Autodesk Inventor part; units mm, degrees
ref_plane "YZ Plane" through (0, 0, 0) normal (1, 0, 0) x (0, 1, 0)
ref_plane "XZ Plane" through (0, 0, 0) normal (0, 1, 0) x (-1, 0, 0)
ref_plane "XY Plane" through (0, 0, 0) normal (0, 0, 1) x (1, 0, 0)
ref_plane "Work Plane1" through (0, 0, 0) normal (0, 0, 1) x (1, 0, 0)
sketch "Sketch1" plane through (0, 0, 0) normal (0, 0, 1) x (1, 0, 0)
  arc A0 (5.9062, 3.651) -> (7.7035, 4.7619) centre (6.8048, 4.2064) ccw
  arc A1 (5.9062, 3.651) -> (2.5768, 6.4477) centre (0, 0) ccw
  arc A2 (3.3608, 8.4097) -> (2.5768, 6.4477) centre (2.9688, 7.4287) ccw
  arc A3 (7.7035, 4.7619) -> (3.3608, 8.4097) centre (0, 0) ccw
  arc A4 (2.5768, -6.4477) -> (3.3608, -8.4097) centre (2.9688, -7.4287) ccw
  arc A5 (2.5768, -6.4477) -> (5.9062, -3.651) centre (0, 0) ccw
  arc A6 (7.7035, -4.7619) -> (5.9062, -3.651) centre (6.8048, -4.2064) ccw
  arc A7 (3.3608, -8.4097) -> (7.7035, -4.7619) centre (0, 0) ccw
  arc A8 (-2.5553, 6.4563) -> (-3.3328, 8.4209) centre (-2.9441, 7.4386) ccw
  arc A9 (-2.5553, 6.4563) -> (-5.9062, 3.651) centre (0, 0) ccw
  arc A10 (-7.7035, 4.7619) -> (-5.9062, 3.651) centre (-6.8048, 4.2064) ccw
  arc A11 (-3.3328, 8.4209) -> (-7.7035, 4.7619) centre (0, 0) ccw
  arc A12 (-5.9062, -3.651) -> (-7.7035, -4.7619) centre (-6.8048, -4.2064) ccw
  arc A13 (-5.9062, -3.651) -> (-2.5553, -6.4563) centre (0, 0) ccw
  arc A14 (-3.3328, -8.4209) -> (-2.5553, -6.4563) centre (-2.9441, -7.4386) ccw
  arc A15 (-7.7035, -4.7619) -> (-3.3328, -8.4209) centre (0, 0) ccw
  circle A16 centre (0.0124, -10.65) radius 1.15
  circle A17 centre (8, 0) radius 1.0564
  circle A18 centre (-8, 0) radius 1.0564
  circle A19 centre (0, 0) radius 5
  circle A20 centre (0, 0) radius 13.7
  line L0 (0, 14.375) -> (-17.375, 14.375)
  line L1 (-17.375, 14.375) -> (-17.375, -14.375)
  line L2 (-17.375, -14.375) -> (0, -14.375)
  circle A21 centre (0, 0) radius 5.15
  arc A22 (5.4809, 3.3881) -> (8.1288, 5.0248) centre (6.8048, 4.2064) ccw
  arc A23 (5.4809, 3.3881) -> (2.3912, 5.9835) centre (0, 0) ccw
  arc A24 (3.5464, 8.874) -> (2.3912, 5.9835) centre (2.9688, 7.4287) ccw
  arc A25 (8.1288, 5.0248) -> (3.5464, 8.874) centre (0, 0) ccw
  arc A26 (8.1288, -5.0248) -> (5.4809, -3.3881) centre (6.8048, -4.2064) ccw
  arc A27 (2.3912, -5.9835) -> (5.4809, -3.3881) centre (0, 0) ccw
  arc A28 (2.3912, -5.9835) -> (3.5464, -8.874) centre (2.9688, -7.4287) ccw
  arc A29 (3.5464, -8.874) -> (8.1288, -5.0248) centre (0, 0) ccw
  circle A30 centre (0.0124, -10.65) radius 1.65
  arc A31 (-5.4809, -3.3881) -> (-2.3713, -5.9914) centre (0, 0) ccw
  arc A32 (-5.4809, -3.3881) -> (-8.1288, -5.0248) centre (-6.8048, -4.2064) ccw
  arc A33 (-8.1288, -5.0248) -> (-3.5168, -8.8858) centre (0, 0) ccw
  arc A34 (-3.5168, -8.8858) -> (-2.3713, -5.9914) centre (-2.9441, -7.4386) ccw
  arc A35 (-2.3713, 5.9914) -> (-5.4809, 3.3881) centre (0, 0) ccw
  arc A36 (-2.3713, 5.9914) -> (-3.5168, 8.8858) centre (-2.9441, 7.4386) ccw
  arc A37 (-3.5168, 8.8858) -> (-8.1288, 5.0248) centre (0, 0) ccw
  arc A38 (-8.1288, 5.0248) -> (-5.4809, 3.3881) centre (-6.8048, 4.2064) ccw
  circle A39 centre (-14.375, -11.375) radius 1.75
  circle A40 centre (-14.375, 11.375) radius 1.75
  arc A41 (0, 13.7) -> (0, -13.7) centre (0, 0) ccw
  line L3 (0, -14.375) -> (0, -13.7)
  line L4 (0, 13.7) -> (0, 14.375)
  line L5 (16.125, 8.6145) -> (16.125, -8.7895)
  line L6 (0, -14.375) -> (16.125, -14.375)
  line L7 (16.125, -14.375) -> (16.125, 14.375)
  line L8 (16.125, 14.375) -> (0, 14.375)
  line L9 (0, 14.375) -> (0, -14.375)
  point P0 (0, 0)
  dimension "d0" = 0.15
  dimension "d1" = 0.5
  dimension "d2" = 0.5
  dimension "d3" = 0.5
  dimension "d4" = 0.5
  dimension "d5" = 0.5
extrude "Extrusion1" add sketch "Sketch1" along normal blind 1.5 contours L9 A21 A20 A30 | A30 L9 A20 A21 | L3 L2 L1 L0 L4 A20 | A20 L4 L8 L7 L5 L6 L3 | A39 | A40
sketch "Sketch2" plane through (0, 0, 1.5) normal (0, 0, 1) x (1, 0, 0)
  line L0 (-17.375, 14.375) -> (-17.375, -14.375)
  line L1 (-17.375, -14.375) -> (16.125, -14.375)
  line L2 (16.125, -14.375) -> (16.125, 14.375)
  line L3 (16.125, 14.375) -> (-17.375, 14.375)
  circle A0 centre (8, 0) radius 1.0564
  circle A1 centre (-8, 0) radius 1.0564
  circle A2 centre (0, 0) radius 5.15
  arc A3 (5.4809, 3.3881) -> (2.3912, 5.9835) centre (0, 0) ccw
  arc A4 (3.5464, 8.874) -> (2.3912, 5.9835) centre (2.9688, 7.4287) ccw
  arc A5 (8.1288, 5.0248) -> (3.5464, 8.874) centre (0, 0) ccw
  arc A6 (5.4809, 3.3881) -> (8.1288, 5.0248) centre (6.8048, 4.2064) ccw
  arc A7 (2.3912, -5.9835) -> (5.4809, -3.3881) centre (0, 0) ccw
  arc A8 (8.1288, -5.0248) -> (5.4809, -3.3881) centre (6.8048, -4.2064) ccw
  arc A9 (3.5464, -8.874) -> (8.1288, -5.0248) centre (0, 0) ccw
  arc A10 (2.3912, -5.9835) -> (3.5464, -8.874) centre (2.9688, -7.4287) ccw
  circle A11 centre (0.0124, -10.65) radius 1.65
  arc A12 (-5.4809, -3.3881) -> (-8.1288, -5.0248) centre (-6.8048, -4.2064) ccw
  arc A13 (-5.4809, -3.3881) -> (-2.3713, -5.9914) centre (0, 0) ccw
  arc A14 (-3.5168, -8.8858) -> (-2.3713, -5.9914) centre (-2.9441, -7.4386) ccw
  arc A15 (-8.1288, -5.0248) -> (-3.5168, -8.8858) centre (0, 0) ccw
  arc A16 (-2.3713, 5.9914) -> (-3.5168, 8.8858) centre (-2.9441, 7.4386) ccw
  arc A17 (-2.3713, 5.9914) -> (-5.4809, 3.3881) centre (0, 0) ccw
  arc A18 (-8.1288, 5.0248) -> (-5.4809, 3.3881) centre (-6.8048, 4.2064) ccw
  arc A19 (-3.5168, 8.8858) -> (-8.1288, 5.0248) centre (0, 0) ccw
  arc A20 (8.1288, -5.0248) -> (5.4809, -3.3881) centre (6.8048, -4.2064) ccw
  line L4 (8.3613, -4.2064) -> (8.3613, -14.375)
  line L5 (-17.375, -14.375) -> (16.125, -14.375)
  arc A21 (-5.4809, -3.3881) -> (-8.1288, -5.0248) centre (-6.8048, -4.2064) ccw
  line L6 (-8.3613, -4.2064) -> (-8.3613, -14.375)
  arc A22 (2.3912, -5.9835) -> (3.5464, -8.874) centre (2.9688, -7.4287) ccw
  line L7 (1.6624, -6.5827) -> (-1.6441, -6.5827)
  arc A23 (-3.5168, -8.8858) -> (-2.3713, -5.9914) centre (-2.9441, -7.4386) ccw
  point P0 (0, 0)
extrude "Extrusion2" add sketch "Sketch2" along normal blind 1.5 contours L3 L2 L1 L4 A8 A7 A10 L7 A14 A13 A12 L6 L0
sketch "Sketch3" plane through (0, 0, 3) normal (0, 0, 1) x (1, 0, 0)
  circle A0 centre (0, 0) radius 6.75
  line L0 (-17.375, -14.375) -> (-8.3613, -14.375)
  line L1 (-8.3613, -14.375) -> (-8.3613, -4.2064)
  arc A1 (-5.4809, -3.3881) -> (-8.3613, -4.2064) centre (-6.8048, -4.2064) ccw
  arc A2 (-5.4809, -3.3881) -> (-2.3713, -5.9914) centre (0, 0) ccw
  arc A3 (-1.6441, -6.5827) -> (-2.3713, -5.9914) centre (-2.9441, -7.4386) ccw
  line L2 (-1.6441, -6.5827) -> (1.6624, -6.5827)
  arc A4 (2.3912, -5.9835) -> (1.6624, -6.5827) centre (2.9688, -7.4287) ccw
  arc A5 (2.3912, -5.9835) -> (5.4809, -3.3881) centre (0, 0) ccw
  arc A6 (8.3613, -4.2064) -> (5.4809, -3.3881) centre (6.8048, -4.2064) ccw
  line L3 (8.3613, -4.2064) -> (8.3613, -14.375)
  line L4 (8.3613, -14.375) -> (16.125, -14.375)
  line L5 (16.125, -14.375) -> (16.125, 14.375)
  line L6 (16.125, 14.375) -> (-17.375, 14.375)
  line L7 (-17.375, 14.375) -> (-17.375, -14.375)
  circle A7 centre (8, 0) radius 1.0564
  circle A8 centre (-8, 0) radius 1.0564
  arc A9 (-2.3713, 5.9914) -> (-5.4809, 3.3881) centre (0, 0) ccw
  arc A10 (-8.1288, 5.0248) -> (-5.4809, 3.3881) centre (-6.8048, 4.2064) ccw
  arc A11 (-3.5168, 8.8858) -> (-8.1288, 5.0248) centre (0, 0) ccw
  arc A12 (-2.3713, 5.9914) -> (-3.5168, 8.8858) centre (-2.9441, 7.4386) ccw
  arc A13 (5.4809, 3.3881) -> (8.1288, 5.0248) centre (6.8048, 4.2064) ccw
  arc A14 (5.4809, 3.3881) -> (2.3912, 5.9835) centre (0, 0) ccw
  arc A15 (3.5464, 8.874) -> (2.3912, 5.9835) centre (2.9688, 7.4287) ccw
  arc A16 (8.1288, 5.0248) -> (3.5464, 8.874) centre (0, 0) ccw
  circle A17 centre (0, 0) radius 5.15
  circle A18 centre (8, 0) radius 2.5
  circle A19 centre (-8, 0) radius 2.5
  line L8 (2.9688, 8.9852) -> (-2.9441, 8.9852)
  line L9 (2.9688, 8.9852) -> (8.8817, 8.9852) construction
  arc A20 (-8.1288, 5.0248) -> (-5.4809, 3.3881) centre (-6.8048, 4.2064) ccw
  line L10 (-8.3613, 4.2064) -> (-8.3613, -4.2064)
  arc A21 (-5.4809, -3.3881) -> (-8.1288, -5.0248) centre (-6.8048, -4.2064) ccw
  arc A22 (5.4809, 3.3881) -> (8.1288, 5.0248) centre (6.8048, 4.2064) ccw
  line L11 (8.3613, 4.2064) -> (8.3613, -4.2064)
  point P0 (0, 0)
  point P1 (-8.3613, -2.4738)
  point P2 (-8.3613, 2.4738)
  point P3 (-2.7693, 8.9852)
  point P4 (8.3613, 2.4738)
  point P5 (8.3613, -2.4738)
  dimension "d10" = 5
  dimension "d11" = 5
  dimension "d12" = 180
extrude "Extrusion3" add sketch "Sketch3" along normal blind 1.5 contours L11 A13 A16 A15 L8 A12 A11 A10 L10 A19 L1 L0 L7 L6 L5 L4 L3 A18
sketch "Sketch4" plane through (0, 0, 4.5) normal (0, 0, 1) x (1, 0, 0)
  line L0 (16.125, -14.375) -> (16.125, 14.375)
  line L1 (-17.375, -14.375) -> (16.125, -14.375)
  line L2 (16.125, 14.375) -> (12.625, 14.375)
  line L3 (12.625, -14.375) -> (16.125, -14.375)
  line L4 (16.125, -14.375) -> (16.125, 14.375)
  circle A0 centre (13.125, 11.375) radius 3
  circle A1 centre (13.125, -11.375) radius 3
  circle A2 centre (-14.375, -11.375) radius 3
  circle A3 centre (-14.375, 11.375) radius 3
  line L5 (-8.3613, -14.375) -> (-8.3613, -2.4738)
  arc A4 (-8.3613, 2.4738) -> (-8.3613, -2.4738) centre (-8, 0) ccw
  line L6 (-8.3613, 2.4738) -> (-8.3613, 4.2064)
  arc A5 (-8.1288, 5.0248) -> (-8.3613, 4.2064) centre (-6.8048, 4.2064) ccw
  arc A6 (-3.5168, 8.8858) -> (-8.1288, 5.0248) centre (0, 0) ccw
  arc A7 (-2.7693, 8.9852) -> (-3.5168, 8.8858) centre (-2.9441, 7.4386) ccw
  line L7 (-2.7693, 8.9852) -> (2.9688, 8.9852)
  arc A8 (3.5464, 8.874) -> (2.9688, 8.9852) centre (2.9688, 7.4287) ccw
  arc A9 (8.1288, 5.0248) -> (3.5464, 8.874) centre (0, 0) ccw
  arc A10 (8.3613, 4.2064) -> (8.1288, 5.0248) centre (6.8048, 4.2064) ccw
  line L8 (8.3613, 4.2064) -> (8.3613, 2.4738)
  arc A11 (8.3613, -2.4738) -> (8.3613, 2.4738) centre (8, 0) ccw
  line L9 (8.3613, -2.4738) -> (8.3613, -14.375)
  line L10 (8.3613, -14.375) -> (16.125, -14.375)
  line L11 (16.125, -14.375) -> (16.125, 14.375)
  line L12 (16.125, 14.375) -> (-17.375, 14.375)
  line L13 (-17.375, 14.375) -> (-17.375, -14.375)
  line L14 (-17.375, -14.375) -> (-8.3613, -14.375)
  point P0 (0, 0)
  dimension "d16" = 6
  dimension "d17" = 6
  dimension "d18" = 6
  dimension "d19" = 6
hole "Hole1" at (-14.375, -11.375, 4.5) at (-14.375, 11.375, 4.5) direction (0, 0, -1) diameter 2.9 end through all countersink diameter 5 countersink angle 90
sketch "Sketch6" plane through (16.125, -14.375, 0) normal (1, 0, 0) x (0, 0, -1)
  line L0 (0, 0) -> (0, 28.75)
  line L1 (0, 28.75) -> (-4.5, 28.75)
  line L2 (-4.5, 0) -> (-4.5, 28.75)
  line L3 (0, 0) -> (-4.5, 0)
  line L4 (0, 28.75) -> (-4.5, 28.75)
  line L5 (-4.5, 28.75) -> (-4.5, 24.25)
  line L6 (-4.5, 24.25) -> (0, 24.25)
  line L7 (0, 24.25) -> (0, 28.75)
  line L8 (0, 0) -> (-4.5, 0)
  line L9 (-4.5, 0) -> (-4.5, 4.5)
  line L10 (-4.5, 4.5) -> (0, 4.5)
  line L11 (0, 4.5) -> (0, 0)
  line L12 (-4.5, 24.25) -> (0, 28.75)
  line L13 (-4.5, 28.75) -> (0, 24.25)
  line L14 (0, 0) -> (-4.5, 0)
  line L15 (0, 4.5) -> (-4.5, 0)
  line L16 (0, 0) -> (-4.5, 4.5)
  point P0 (0, 14.375)
  point P1 (-2.25, 26.5)
  point P2 (-2.25, 2.25)
  dimension "d34" = 4.5
  dimension "d35" = 4.5
  dimension "d36" = 4.5
  dimension "d37" = 4.5
hole "Hole3" at (16.125, 12.125, 2.25) at (16.125, -12.125, 2.25) direction (-1, 0, 0) diameter 3 depth 3.5 counterbore diameter 3.5 counterbore depth 1.5
properties part number "right_motor_front_mount" material "Nylon 6/6"
Check sheet for the modelled part. Datum: model origin and axes. Units: mm. A direction names the side the tool comes from. Give positions to 0.01 mm unless a question says otherwise; leave off trailing zeros. Write each loop counter-clockwise with the first axis right and the second up, starting at its lowest first coordinate (ties: lowest second). Pieces come first, ordered by that corner, then holes. Notation, with made-up numbers: M 70.5,24 L 121.5,24 A18 ccw 121.5,41 Z; hole C 22,9.25 d6. An arc over 180 degrees is marked long. Use one line per item in the form item = value.
(1) Section check B-B on x = 0. Record the boundary of the cut face in (y, z) (3 decimals).
Answer block:
outline = M -14.375,0 L -12.3,0 L -12.3,1.5 L -14.375,1.5 Z; M -9,0 L -5.15,0 L -5.15,3 L -6.583,3 L -6.583,1.5 L -9,1.5 Z; M 5.15,0 L 14.375,0 L 14.375,4.5 L 8.985,4.5 L 8.985,3 L 5.15,3 Z
(2) Section check C-C on z = 2.25. State how many separate pieces and enclosed holes the cut face has, plus the area to 3 significant figures.
Answer block:
separate_pieces = 1
enclosed_holes = 7
area = 628 mm2
(3) Draft check along Z on faces 1 (the cylindrical face through (15.36, -13.86, 2.48)), 2 (the flat face through (-2, 5, 3)), 3 (the flat face through (16.125, 0, 2)). Enter one of: pulls with the +Z half, pulls with the -Z half, needs draft (parallel to the pull), parting line crosses it, or undercut.
Answer block:
face_1 = undercut
face_2 = pulls with the +Z half
face_3 = needs draft
(4) Material ranges on line 1 along Y through (x, z) = (-14.5, 1.35) (3 decimals); line 2 along X through (y, z) = (-11.5, 3.2) (3 decimals); line 3 along X through (y, z) = (-7.75, 2.95) (3 decimals), recorded low to high.
Answer block:
line_1 = -14.375 to -12.82, -9.93 to 9.93, 12.82 to 14.375
line_2 = -17.375 to -15.82, -12.93 to -8.361, 8.361 to 12.625
line_3 = -17.375 to -8.361, 8.361 to 16.125
(5) Section check A-A on y = 0. Record the boundary of the cut face in (x, z) (3 decimals), plus the area to 3 significant figures.
Answer block:
outline = M -17.375,0 L -9.056,0 L -9.056,3 L -10.5,3 L -10.5,4.5 L -17.375,4.5 Z; M -6.944,0 L -5.15,0 L -5.15,3 L -6.944,3 Z; M 5.15,0 L 6.944,0 L 6.944,3 L 5.15,3 Z; M 9.056,0 L 16.125,0 L 16.125,4.5 L 10.5,4.5 L 10.5,3 L 9.056,3 Z
area = 75.7 mm2
(6) Tool access check on faces 4 (the cylindrical face through (-10.5, 0, 3.7)), 5 (the cylindrical face through (13.611, 12.7, 0.864)), 6 (the cylindrical face through (-6.17, 7.3, 2.22)), 7 (the flat face through (0, 14.375, 2)), 8 (the flat face through (0, 8.985, 4)). Record the directions out of +Z, -Z, +X, -X, +Y, -Y that give a thin tool (end or side, any length) a straight path to the whole face; none if there is none.
Answer block:
face_4 = +Z
face_5 = +X
face_6 = +Z, -Z
face_7 = +Z, -Z, +X, -X, +Y
face_8 = +Z, -Y
(7) Depth check by flat-ended pin: P1, Ø1.7, axis at x = -14.375, y = 11.375, coming from the +Z side; P2, Ø0.8, axis at x = -0.5, z = 4, coming from the -Y side; P3, Ø3, axis at x = -6.5, y = -1.5, coming from the +Z side; P4, Ø2.5, axis at y = 12.5, z = 2, coming from the +X side (3 decimals). Enter the tip coordinate at first touch or a pass-through.
Answer block:
P1 = through
P2 = 8.99
P3 = 3
P4 = 14.625
